Here's how the part is built. I have some questions about the finished solid (model axes, mm). A direction names the side the tool comes from. Coordinates: 2 decimals unless noted, no trailing zeros. Write each loop counter-clockwise with the first axis right and the second up, starting at its lowest first coordinate (ties: lowest second). Pieces come first, ordered by that corner, then holes.
Item 1: Please list where these lines run through material, in increasing order: line 1 (Z direction, x = -33.5, y = -4); line 2 (X direction, y = -3, z = 10.5); line 3 (X direction, y = -4.75, z = -5).
Item 2: I want a section at C-C (x = -2). Please give me the cut outline in (y, z).
Item 3: For faces 1 (the face through (-29, -5, 50)), 2 (the face through (-4, -5, 50)), 3 (the face through (-41, -5, 20.5)), 4 (the face through (-5, -5, 0)), which set-ups out of +Z, -Z, +X, -X, +Y, -Y let a thin tool reach every point of the face, with its end or its side?
Item 4: I'm going to push flat-ended pins straight in: P1, Ø5, axis at y = -5, z = 43, coming from the -X side; P2, Ø5, axis at x = -27, y = -5, coming from the -Z side; P3, Ø1.5, axis at x = 3.5, y = -3, coming from the +Z side. Where does each tip first touch, or does it pass through?
Item 5: I want a section at B-B (z = 51.5). Please give me the cut outline in (x, y).
Item 6: I want a section at A-A (y = -4). Please give me the cut outline in (x, z).
from build123d import *

# Parameters (mm, degrees)
F0_W     = 9
F0_H     = 9
F1_DEPTH = 10


with BuildPart() as f1:
    # F0 (on Front) → F1 (new body)
    with BuildSketch(Plane.XZ):
        Polygon((-21.18931, 50), (-36.68931, 50), (-36.68931, 29.5), (-36.68931, 20.5), (-36.68931, 0), (-21.18931, 0), (-12.18931, 0), (3.31069, 0), (3.31069, 20.5), (3.31069, 29.5), (3.31069, 50), (-12.18931, 50), align=None)
        with Locations((-16.68931, 54.5)):
            Rectangle(F0_W, F0_H)
        with Locations((-41.18931, 25)):
            Rectangle(F0_W, F0_H)
        with Locations((7.81069, 25)):
            Rectangle(F0_W, F0_H)
        with Locations((-16.68931, -4.5)):
            Rectangle(F0_W, F0_H)
    extrude(amount=F1_DEPTH)


solid = f1.part
Answer:
1. line 1: z = 0 to 50
1. line 2: x = -36.69 to 3.31
1. line 3: x = -21.19 to -12.19
2. outline: (-10, 0) - (0, 0) - (0, 50) - (-10, 50) - close
3. face 1: +Z, -X, +Y, -Y
3. face 2: +Z, +X, +Y, -Y
3. face 3: -Z, -X, +Y, -Y
3. face 4: -Z, +X, +Y, -Y
4. P1: stops at x = -36.69
4. P2: stops at z = 0
4. P3: stops at z = 50
5. outline: (-21.19, -10) - (-12.19, -10) - (-12.19, 0) - (-21.19, 0) - close
6. outline: (-45.69, 20.5) - (-36.69, 20.5) - (-36.69, 0) - (-21.19, 0) - (-21.19, -9) - (-12.19, -9) - (-12.19, 0) - (3.31, 0) - (3.31, 20.5) - (12.31, 20.5) - (12.31, 29.5) - (3.31, 29.5) - (3.31, 50) - (-12.19, 50) - (-12.19, 59) - (-21.19, 59) - (-21.19, 50) - (-36.69, 50) - (-36.69, 29.5) - (-45.69, 29.5) - close
